```python
from build123d import *

# Parameters (mm, degrees)
ESBO_O1_W                = 200
ESBO_O1_H                = 200
RESSALTO_EXTRUS_O1_DEPTH = 50
CORTE_EXTRUS_O1_DEPTH    = 7


with BuildPart() as part:
    # Esboço1 → Ressalto-extrusão1 (new body)
    with BuildSketch(Plane.XY):
        with Locations((100, 100)):
            Rectangle(ESBO_O1_W, ESBO_O1_H)
    extrude(amount=RESSALTO_EXTRUS_O1_DEPTH)

    # Esboço3 → Corte-extrusão1 (cut)
    with BuildSketch(Plane(origin=(0, 0, 0), x_dir=(-1, 0, 0), z_dir=(0, 0, -1))):
        Polygon((-160.5, 176.55), (-160.5, 177.05), (-160.5, 178.95), (-179.5, 178.95), (-179.5, 177.05), (-179.5, 176.55), (-179.5, 174.65), (-160.5, 174.65), align=None)
        Polygon((-39.5, 177.05), (-39.5, 178.95), (-20.5, 178.95), (-20.5, 177.05), (-20.5, 176.55), (-20.5, 174.65), (-39.5, 174.65), (-39.5, 176.55), align=None)
        Polygon((-39.5, 23.45), (-39.5, 22.95), (-39.5, 21.05), (-20.5, 21.05), (-20.5, 22.95), (-20.5, 23.45), (-20.5, 25.35), (-39.5, 25.35), align=None)
        Polygon((-160.5, 22.95), (-160.5, 21.05), (-179.5, 21.05), (-179.5, 22.95), (-179.5, 23.45), (-179.5, 25.35), (-160.5, 25.35), (-160.5, 23.45), align=None)
    extrude(amount=-CORTE_EXTRUS_O1_DEPTH, mode=Mode.SUBTRACT)


solid = part.part
```
Work out the finished part from the listing and answer in its coordinate system (mm). A direction names the side the tool comes from. Give positions to 0.01 mm unless a question says otherwise; leave off trailing zeros. Use CSV: the item, a comma, the result in double quotes. Start each with the question number.
(1) A tool of negligible diameter and unlimited length cuts with its end or side. For faces 4 (the face through (30, 178.95, 3)), 5 (the face through (0, 99, 25)), from which of +Z, -Z, +X, -X, +Y, -Y can it reach the whole face along a straight path? Write none if from no direction.
(2) This flat-tipped pin is pushed along its axis until it touches: pin 1 (3.5 mm diameter, centred on x = 170, y = 23.5, fed in from -Z). Where does it stop, or does it pass through?
(3) Determine the mould class of faces 1 (the face through (200, 99, 25)), 2 (the face through (170, 174.65, 3)), 3 (the face through (99, 101, 50)) for opening direction X: released by +X, released by -X, zero draft, split by the parting line, or undercut.
Results found:
1,face 4,"-Z"
1,face 5,"+Z, -Z, -X, +Y, -Y"
2,pin 1,"z = 7"
3,face 1,"released by +X"
3,face 2,"undercut"
3,face 3,"zero draft"
